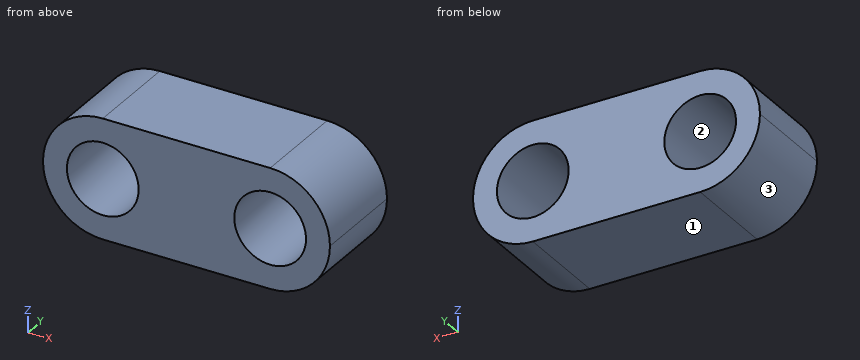
```python
from build123d import *

# Parameters (mm, degrees)
SKETCH1_W           = 12
SKETCH1_H           = 5
BOSS_EXTRUDE1_DEPTH = 4
SKETCH2_R           = 1.5
CUT_EXTRUDE1_DEPTH  = 4
SKETCH3_R           = 1.5
CUT_EXTRUDE2_DEPTH  = 4
FILLET1_R           = 2.5


with BuildPart() as part:
    # Sketch1 → Boss-Extrude1 (new body)
    with BuildSketch(Plane(origin=(0, 0, 0), x_dir=(1, 0, 0), z_dir=(0, 1, 0))):
        Rectangle(SKETCH1_W, SKETCH1_H)
    extrude(amount=BOSS_EXTRUDE1_DEPTH)

    # Sketch2 → Cut-Extrude1 (cut)
    with BuildSketch(Plane(origin=(0, 4, 0), x_dir=(1, 0, 0), z_dir=(0, 1, 0))):
        with Locations(Location((3.5, 0, 0), (0, 0, 270))):
            Circle(SKETCH2_R)
    extrude(amount=-CUT_EXTRUDE1_DEPTH, mode=Mode.SUBTRACT)

    # Sketch3 → Cut-Extrude2 (cut)
    with BuildSketch(Plane(origin=(0, 4, 0), x_dir=(1, 0, 0), z_dir=(0, 1, 0))):
        with Locations(Location((-3.5, 0, 0), (0, 0, 270))):
            Circle(SKETCH3_R)
    extrude(amount=-CUT_EXTRUDE2_DEPTH, mode=Mode.SUBTRACT)

    # Fillet1
    fillet1_edges = [part.edges().sort_by_distance(p)[0] for p in [
        (6, 2, 2.5),
        (6, 2, -2.5),
        (-6, 2, 2.5),
        (-6, 2, -2.5),
    ]]
    fillet(fillet1_edges, radius=FILLET1_R - 0.0001)  # a hair under: the kernel refuses the full size


solid = part.part
```
Part model, mm, in its own coordinate system. Face numbers are marked on the shaded views. Give positions to 0.01 mm unless a question says otherwise; leave off trailing zeros. Loops run counter-clockwise (first coordinate to the right, second up) from the corner with the lowest first, then second, coordinate; pieces in that order, holes last. Notation, with made-up numbers: M 51,52.5 L 84,52.5 A27 cw 84,73.5 Z; hole C 68,83.5 d11. An arc over 180 degrees is marked long. Return JSON: item names as keys, results as strings.
1) Saw through at A-A, the plane y = 3.7. Count the separate pieces of the cut face and the enclosed holes in it, then the cut area to 3 significant figures.
Calculated:
{"separate pieces": "1", "enclosed holes": "2", "area": "40.5 mm2"}
2) Drill centre lines: line 1 (X direction, y = 1.2, z = 0); line 2 (X direction, y = 2.2, z = 1.15); line 3 (Z direction, x = -2.5, y = 0.8). Where is each one in solid material? Low to high.
Calculated:
{"line 1": "x = -6 to -5, -2 to 2, 5 to 6", "line 2": "x = -5.72 to -4.46, -2.54 to 2.54, 4.46 to 5.72", "line 3": "z = -2.5 to -1.12, 1.12 to 2.5"}
3) Flat gauge pins, fed straight in: pin 1 Ø1.5 at (y, z) = (0.5, -1.5) entering from +X; pin 2 Ø3 at (x, z) = (-3.5, -1) entering from +Y; pin 3 Ø1.8 at (x, z) = (3.5, 0) entering from -Y. Where does each tip first touch, or does it go through?
Calculated:
{"pin 1": "stops at x = 5.88", "pin 2": "stops at y = 4", "pin 3": "passes through"}
4) Saw through at B-B, the plane z = -0.7. List the corners of the cut face in (x, y), then the cut area to 3 significant figures.
Calculated:
{"outline": "M -5.9,0 L -4.83,0 L -4.83,4 L -5.9,4 Z; M -2.17,0 L 2.17,0 L 2.17,4 L -2.17,4 Z; M 4.83,0 L 5.9,0 L 5.9,4 L 4.83,4 Z", "area": "26.0 mm2"}
5) Saw through at D-D, the plane z = -1.65. List the corners of the cut face in (x, y), then the cut area to 3 significant figures.
Calculated:
{"outline": "M -5.38,0 L 5.38,0 L 5.38,4 L -5.38,4 Z", "area": "43.0 mm2"}
6) Saw through at C-C, the plane z = 0.75. List the corners of the cut face in (x, y).
Calculated:
{"outline": "M -5.88,0 L -4.8,0 L -4.8,4 L -5.88,4 Z; M -2.2,0 L 2.2,0 L 2.2,4 L -2.2,4 Z; M 4.8,0 L 5.88,0 L 5.88,4 L 4.8,4 Z"}
7) Pull direction X, two halves, no side cores. Call the marked faces 1, 2 and 3: released by +X, released by -X, zero draft, split by the parting line, or undercut.
Calculated:
{"face 1": "zero draft", "face 2": "undercut", "face 3": "released by -X"}
